from build123d import *

# Parameters (mm, degrees)
SKETCH1_W            = 55.5
SKETCH1_H            = 40.4
BASE_DEPTH           = 5
SKETCH2_W            = 55.5
SKETCH2_H            = 25.5
WALL_DEPTH           = 5
SKETCH3_W            = 7
SKETCH3_H            = 20.5
MOUNTINGTABS_DEPTH   = 5
LIPS_REACH           = 75.23
SKETCH5_R            = 2.125
MOUNTINGHOLES_DEPTH  = 5
FILLETS_R            = 3.5
SKETCH6_R            = 2.125
THROUGHHOLE_DEPTH    = 5
FILLETS_OF_MIRROR3_R = 3.5
SKETCH7_W            = 104.516790574
SKETCH7_H            = 66.327963249
CUT_EXTRUDE1_DEPTH   = 73
SKETCH8_R            = 2.125
BOSS_EXTRUDE1_DEPTH  = 5


with BuildPart() as part:
    # Sketch1 → base (new body)
    with BuildSketch(Plane(origin=(0, 0, 0), x_dir=(1, 0, 0), z_dir=(0, 1, 0))):
        with Locations((27.75, 20.2)):
            Rectangle(SKETCH1_W, SKETCH1_H)
    base = extrude(amount=BASE_DEPTH)

    # Sketch2 → wall (add)
    with BuildSketch(Plane(origin=(0, 0, -40.4), x_dir=(-1, 0, 0), z_dir=(0, 0, -1))):
        with Locations((-27.75, 12.75)):
            Rectangle(SKETCH2_W, SKETCH2_H)
    wall = extrude(amount=-WALL_DEPTH)

    # Sketch3 → mountingTabs (add)
    with BuildSketch(Plane.XY.offset(-8.2)):
        with Locations((3.5, 15.25)):
            Rectangle(SKETCH3_W, SKETCH3_H)
        with Locations((52, 15.25)):
            Rectangle(SKETCH3_W, SKETCH3_H)
    mountingtabs = extrude(amount=MOUNTINGTABS_DEPTH)

    # lips: up to this face of the body (flat: up to its plane)
    lips_end = Plane(part.part.faces().sort_by_distance((27.75, 12.75, -40.4))[0])
    # Sketch4 → lips (add, up to the picked face)
    with BuildSketch(Plane.XY, mode=Mode.PRIVATE) as lips_sk1:
        with BuildLine():
            Line((0, 0), (-10.208884478, 7.148337868))
            ThreePointArc((-10.208884478, 7.148337868), (-11.894564223, 9.792816133), (-11.218174515, 12.85505036))
            Line((-11.218174515, 12.85505036), (0, 5))
            Line((0, 5), (0, 0))
        make_face()
    lips_tool1 = split(extrude(lips_sk1.sketch, amount=-LIPS_REACH, mode=Mode.PRIVATE), bisect_by=lips_end, keep=Keep.BOTH, mode=Mode.PRIVATE)
    # Sketch4 → lips (add, up to the picked face)
    with BuildSketch(Plane.XY, mode=Mode.PRIVATE) as lips_sk2:
        with BuildLine():
            Line((55.5, 5), (66.718174515, 12.85505036))
            ThreePointArc((66.718174515, 12.85505036), (67.394564223, 9.792816133), (65.708884478, 7.148337868))
            Line((65.708884478, 7.148337868), (55.5, 0))
            Line((55.5, 0), (55.5, 5))
        make_face()
    lips_tool2 = split(extrude(lips_sk2.sketch, amount=-LIPS_REACH, mode=Mode.PRIVATE), bisect_by=lips_end, keep=Keep.BOTH, mode=Mode.PRIVATE)
    lips_1 = lips_tool1.solids().sort_by(Axis((-5.839287, 6.590277, 0), (0, 0, -1)))[0]
    add(lips_1)
    lips_2 = lips_tool2.solids().sort_by(Axis((61.339287, 6.590277, 0), (0, 0, -1)))[0]
    add(lips_2)
    lips = lips_1 + lips_2  # lips as one shape, for the pattern or mirror that repeats it

    # Sketch5 → mountingHoles (cut)
    with BuildSketch(Plane.XY.offset(-3.2)):
        with Locations((3.75, 20.25)):
            Circle(SKETCH5_R)
        with Locations(Location((3.75, 10.25, 0), (0, 0, 180))):
            Circle(SKETCH5_R)
        with Locations((51.75, 10.25)):
            Circle(SKETCH5_R)
        with Locations(Location((51.75, 20.25, 0), (0, 0, 180))):
            Circle(SKETCH5_R)
    mountingholes = extrude(amount=-MOUNTINGHOLES_DEPTH, mode=Mode.SUBTRACT)

    # fillets
    fillets_edges = [part.edges().sort_by_distance(p)[0] for p in [
        (0, 25.5, -37.9),
        (55.5, 25.5, -37.9),
        (0, 25.5, -5.7),
        (55.5, 25.5, -5.7),
    ]]
    fillet(fillets_edges, radius=FILLETS_R)

    # Sketch6 → throughHole (cut)
    with BuildSketch(Plane.XY.offset(-35.4)):
        with Locations((38.25, 15.25)):
            Circle(SKETCH6_R)
    throughhole = extrude(amount=-THROUGHHOLE_DEPTH, mode=Mode.SUBTRACT)

    # Mirror3: base, wall, mountingTabs, lips, mountingHoles, throughHole across plane
    add(base.mirror(Plane.XY))
    add(wall.mirror(Plane.XY))
    add(mountingtabs.mirror(Plane.XY))
    add(lips.mirror(Plane.XY))
    add(mountingholes.mirror(Plane.XY), mode=Mode.SUBTRACT)
    add(throughhole.mirror(Plane.XY), mode=Mode.SUBTRACT)

    # fillets of Mirror3
    fillets_of_mirror3_edges = [part.edges().sort_by_distance(p)[0] for p in [
        (0, 25.5, 37.9),
        (55.5, 25.5, 37.9),
        (0, 25.5, 5.7),
        (55.5, 25.5, 5.7),
    ]]
    fillet(fillets_of_mirror3_edges, radius=FILLETS_OF_MIRROR3_R)

    # Sketch7 → Cut-Extrude1 (cut)
    with BuildSketch(Plane.XY):
        with Locations((25.489671827, 15.622702088)):
            Rectangle(SKETCH7_W, SKETCH7_H)
    extrude(amount=-CUT_EXTRUDE1_DEPTH, mode=Mode.SUBTRACT)

    # Sketch8 → Boss-Extrude1 (add)
    # profile 1 of 2: a face of its own
    with BuildSketch(Plane.XY.offset(8.2)):
        with BuildLine():
            Line((7, 25.5), (3.5, 25.5))
            ThreePointArc((3.5, 25.5), (1.025126266, 24.474873734), (0, 22))
            Line((0, 22), (0, 5))
            Line((0, 5), (7, 5))
            Line((7, 5), (7, 25.5))
        make_face()
        with Locations((3.75, 20.25)):
            Circle(SKETCH8_R, mode=Mode.SUBTRACT)
        with Locations(Location((3.75, 10.25, 0), (0, 0, 180))):
            Circle(SKETCH8_R, mode=Mode.SUBTRACT)
    # profile 2 of 2: a face of its own
    with BuildSketch(Plane.XY.offset(8.2)):
        with BuildLine():
            Line((55.5, 5), (55.5, 22))
            ThreePointArc((55.5, 22), (54.474873734, 24.474873734), (52, 25.5))
            Line((52, 25.5), (48.5, 25.5))
            Line((48.5, 25.5), (48.5, 5))
            Line((48.5, 5), (55.5, 5))
        make_face()
        with Locations(Location((51.75, 20.25, 0), (0, 0, 180))):
            Circle(SKETCH8_R, mode=Mode.SUBTRACT)
        with Locations((51.75, 10.25)):
            Circle(SKETCH8_R, mode=Mode.SUBTRACT)
    extrude(amount=BOSS_EXTRUDE1_DEPTH)


solid = part.part
Could you check a few things on this model? Use its own coordinates, in mm. A direction names the side the tool comes from. Give positions to 0.01 mm unless a question says otherwise; leave off trailing zeros. Write each loop counter-clockwise with the first axis right and the second up, starting at its lowest first coordinate (ties: lowest second). Pieces come first, ordered by that corner, then holes. Notation, with made-up numbers: (-29.75, 38.5) -> (2.25, 38.5) arc R19 ccw to (2.25, 45.5) -> close; hole circle Ø7 at (-33.75, 11). An arc over 180 degrees is marked (long way). Answer as CSV lines item,"result". Start each with the question number.
(1) I'm going to push flat-ended pins straight in: pin 1 Ø3.5 at (x, y) = (52.5, 16) entering from -Z; pin 2 Ø2.5 at (y, z) = (16, 38.5) entering from +X; pin 3 Ø3 at (x, z) = (-2, 9.5) entering from +Y. Where does each tip first touch, or does it pass through?
(2) Please list where these lines run through material, in increasing order: line 1 (Y direction, x = 51.75, z = 5.75) (3 decimals); line 2 (Z direction, x = 29, y = 17); line 3 (Y direction, x = 7, z = 26).
(3) If we section it at C-C, the plane z = 6: Write out the boundary of the cut face in (x, y) (3 decimals).
(4) If we section it at D-D, the plane y = 10.25: Write out the boundary of the cut face in (x, z) (3 decimals).
(5) If we section it at B-B, the plane z = 37.5: Write out the boundary of the cut face in (x, y) (3 decimals).
(6) Which directions (+Z, -Z, +X, -X, +Y, -Y) give clear straight access to the entire face, cutting with the end or side of a thin tool? Please do faces 1 (the face through (49.627, 10.343, 8.13)), 2 (the face through (61.03, 8.87, 20.48)), 3 (the face through (48.5, 15, 8)), 4 (the face through (40.213, 14.436, 37.865)), 5 (the face through (52, 15, 13.2)).
(7) If we mould it in two halves opening along Y, with no side actions, what happens to faces 6 (the face through (-5.688, 8.983, 19.917)), 7 (the face through (2.06, 18.96, 8.13)), 8 (the face through (28, 15, 35.4))? For each: +Y half, -Y half, draft (parallel to the pull), parting line (faces both ways), or undercut.
(8) If we section it at A-A, the plane y = 20.25: Write out the boundary of the cut face in (x, z) (3 decimals), and give its area (4 significant figures).
Answer list:
1,pin 1,"z = 3.2"
1,pin 2,"x = 55.5"
1,pin 3,"y = 7.45"
2,line 1,"0 to 8.125, 12.375 to 18.125, 22.375 to 25.5"
2,line 2,"35.4 to 40.4"
2,line 3,"0 to 5"
3,outline,"(-11.218, 12.855) arc R4.1 ccw to (-10.209, 7.148) -> (0, 0) -> (55.5, 0) -> (65.709, 7.148) arc R4.1 ccw to (66.718, 12.855) -> (55.5, 5) -> (55.5, 22) arc R3.5 ccw to (52, 25.5) -> (48.5, 25.5) -> (48.5, 5) -> (7, 5) -> (7, 25.5) -> (3.5, 25.5) arc R3.5 ccw to (0, 22) -> (0, 5) -> close; hole circle Ø4.25 at (3.75, 10.25); hole circle Ø4.25 at (3.75, 20.25); hole circle Ø4.25 at (51.75, 10.25); hole circle Ø4.25 at (51.75, 20.25)"
4,outline,"(-11.949, 0) -> (-7.498, 0) -> (-7.498, 40.4) -> (-11.949, 40.4) -> close; (0, 3.2) -> (1.625, 3.2) -> (1.625, 13.2) -> (0, 13.2) -> close; (0, 35.4) -> (55.5, 35.4) -> (55.5, 40.4) -> (0, 40.4) -> close; (5.875, 3.2) -> (7, 3.2) -> (7, 13.2) -> (5.875, 13.2) -> close; (48.5, 3.2) -> (49.625, 3.2) -> (49.625, 13.2) -> (48.5, 13.2) -> close; (53.875, 3.2) -> (55.5, 3.2) -> (55.5, 13.2) -> (53.875, 13.2) -> close; (62.998, 0) -> (67.449, 0) -> (67.449, 40.4) -> (62.998, 40.4) -> close"
5,outline,"(-11.218, 12.855) arc R4.1 ccw to (-10.209, 7.148) -> (0, 0) -> (55.5, 0) -> (65.709, 7.148) arc R4.1 ccw to (66.718, 12.855) -> (55.5, 5) -> (55.5, 22) arc R3.5 ccw to (52, 25.5) -> (3.5, 25.5) arc R3.5 ccw to (0, 22) -> (0, 5) -> close; hole circle Ø4.25 at (38.25, 15.25)"
6,face 1,"-Z"
6,face 2,"+Z, -Z, +Y"
6,face 3,"-Z, +Y"
6,face 4,"+Z, -Z"
6,face 5,"+Y"
7,face 6,"+Y half"
7,face 7,"undercut"
7,face 8,"draft"
8,outline,"(0, 3.2) -> (1.625, 3.2) -> (1.625, 13.2) -> (0, 13.2) -> close; (0, 35.4) -> (55.5, 35.4) -> (55.5, 40.4) -> (0, 40.4) -> close; (5.875, 3.2) -> (7, 3.2) -> (7, 13.2) -> (5.875, 13.2) -> close; (48.5, 3.2) -> (49.625, 3.2) -> (49.625, 13.2) -> (48.5, 13.2) -> close; (53.875, 3.2) -> (55.5, 3.2) -> (55.5, 13.2) -> (53.875, 13.2) -> close"
8,area,"332.5 mm^2"
